Geometry: see drawing. Coordinates: mm, zero at the bounding-box minimum. A direction names the side the tool comes from. Coordinates: 2 decimals unless noted, no trailing zeros. Loops run counter-clockwise (first coordinate to the right, second up) from the corner with the lowest first, then second, coordinate; pieces in that order, holes last. Notation, with made-up numbers: (76, 5) -> (123, 5) arc R12 ccw to (123, 19) -> close; hole circle Ø2 at (77, 54.25). An arc over 180 degrees is marked (long way). One line per item, written item: value. Start each with the question number.
Item 1: Section query D-D on x = 66. Return loops of the section in (y, z), then the cut area to 3 significant figures.
Item 2: Ray query, probe 1 along Y at (x, z) = (53.5, 8.75); probe 2 along X at (y, z) = (88, 8); probe 3 along X at (y, z) = (24.5, 20). Return the intervals inside material, ascending. Write a range as from..to.
Item 3: Section query C-C on z = 16.5. Return loops of the section in (x, y).
Item 4: Mould query, pull axis X, two halves, no side actions, for the marked faces 1, 2, 3 and 4. Classes: +X half, -X half, draft (parallel to the pull), parting line (faces both ways), or undercut.
Item 5: Section query B-B on y = 88.5. Return loops of the section in (x, z), then the cut area to 3 significant figures.
Item 6: Section query A-A on x = 53.5. Return loops of the section in (y, z), then the cut area to 3 significant figures.
Item 7: Set-up query: the marked faces 5 and 6. Return all of +Z, -Z, +X, -X, +Y, -Y with unobstructed straight access to the full face (end or side cutting, diameter ignored); none if empty.
Item 8: Contact query for flat-ended pins moving along their axis: pin 1 Ø15 at (y, z) = (16.5, 17) entering from -X; pin 2 Ø3 at (x, z) = (24.5, 14.5) entering from +Y; pin 3 Ø5 at (x, z) = (45, 24) entering from +Y. Output: stop coordinate, or through.
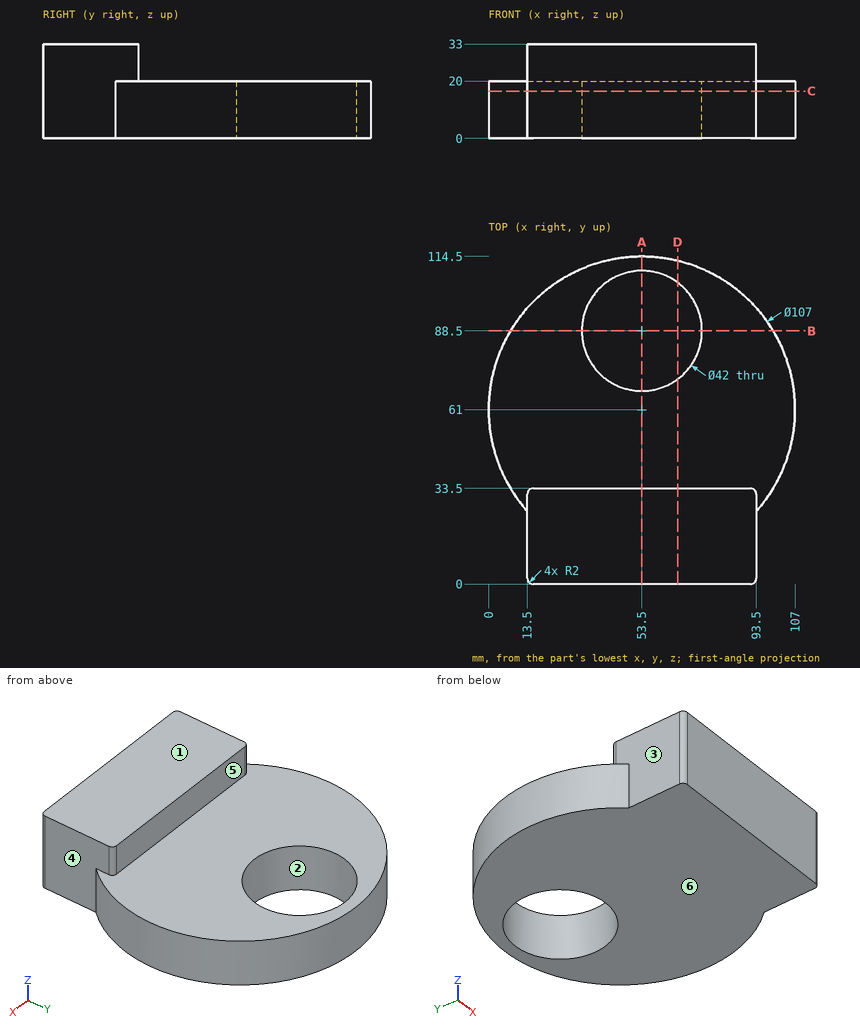
Reply:
1. outline: (0, 0) -> (71.63, 0) -> (71.63, 20) -> (33.5, 20) -> (33.5, 33) -> (0, 33) -> close; (105.37, 0) -> (113.02, 0) -> (113.02, 20) -> (105.37, 20) -> close
1. area: 2,020 mm²
2. probe 1: y = 0..67.5, 109.5..114.5
2. probe 2: x = 7.31..32.51, 74.49..99.69
2. probe 3: x = 13.5..93.5
3. outline: (13.5, 2) arc R2 ccw to (15.5, 0) -> (91.5, 0) arc R2 ccw to (93.5, 2) -> (93.5, 25.47) arc R53.5 ccw (long way) to (13.5, 25.47) -> close; hole circle Ø42 at (53.5, 88.5)
4. face 1: draft
4. face 2: undercut
4. face 3: -X half
4. face 4: +X half
5. outline: (7.61, 0) -> (32.5, 0) -> (32.5, 20) -> (7.61, 20) -> close; (74.5, 0) -> (99.39, 0) -> (99.39, 20) -> (74.5, 20) -> close
5. area: 996 mm²
6. outline: (0, 0) -> (67.5, 0) -> (67.5, 20) -> (33.5, 20) -> (33.5, 33) -> (0, 33) -> close; (109.5, 0) -> (114.5, 0) -> (114.5, 20) -> (109.5, 20) -> close
6. area: 1,890 mm²
7. face 5: +Z, +X, -X, +Y
7. face 6: -Z, +X, -X, +Y, -Y
8. pin 1: stops at x = 13.5
8. pin 2: stops at y = 106.89
8. pin 3: stops at y = 33.5
